Geometry: final body of the model. Coordinates: model frame, mm. Coordinates: 2 decimals unless noted, no trailing zeros. Order: outer loops, then holes, each group sorted by start corner. A loop starts at its lowest first (then second) coordinate and runs counter-clockwise, first axis right, second up. Notation, with made-up numbers: (-31, -37) -> (1, -37) arc R14 ccw to (1, -11) -> close; hole circle Ø8 at (75.25, 87). An arc over 180 degrees is marked (long way). Answer in a Markdown table with one row per item. Add a question column.
1) Section query B-B on z = -451. Return the cut outline in (x, y).
2) Ray query, line 1 (X direction, y = 12, z = -18); line 2 (X direction, y = 20.2, z = -280); line 3 (Z direction, x = 232, y = 8.75). Return the intervals inside material, ascending. Write a range as from..to.
3) Contact query for flat-ended pins moving along their axis: P1, Ø1.5, axis at y = 6, z = -223.5, coming from the -X side; P2, Ø1.5, axis at y = 6.5, z = 164.5, coming from the +X side; P3, Ø1.5, axis at y = 12.5, z = -389.5, coming from the -X side. Output: stop coordinate, or through.
4) Section query A-A on x = -241. Return the cut outline in (y, z), then the cut area to 3 significant figures.
```python
from build123d import *

# Parameters (mm, degrees)
ESQUISSE1_R             = 600
BOSS_EXTRU_1_DEPTH      = 22
ESQUISSE2_R             = 4
ENL_V_MAT_EXTRU_1_DEPTH = 23
ENL_V_MAT_EXTRU_2_DEPTH = 8
ESQUISSE4_R             = 12
ENL_V_MAT_EXTRU_3_DEPTH = 5
ESQUISSE6_R             = 3
ENL_V_MAT_EXTRU_4_DEPTH = 23


with BuildPart() as part:
    # Esquisse1 → Boss.-Extru.1 (new body)
    with BuildSketch(Plane(origin=(0, 0, 0), x_dir=(1, 0, 0), z_dir=(0, 1, 0))):
        with Locations(Location((0, 0, 0), (0, 0, 270))):  # turned: the seam where the file's is
            Circle(ESQUISSE1_R)
    extrude(amount=BOSS_EXTRU_1_DEPTH)

    # Esquisse2 → Enlèv. mat.-Extru.1 (cut, through all)
    with BuildSketch(Plane(origin=(0, 22, 0), x_dir=(1, 0, 0), z_dir=(0, 1, 0))):
        with Locations(Location((0, 280, 0), (0, 0, 270))):  # turned: the seam where the file's is
            Circle(ESQUISSE2_R)
    extrude(amount=-ENL_V_MAT_EXTRU_1_DEPTH, mode=Mode.SUBTRACT)

    # Esquisse3 → Enlèv. mat.-Extru.2 (cut)
    with BuildSketch(Plane.XZ):
        Polygon((6.5, -280), (6.5, -276.24722325), (3.25, -274.370834875), (0, -272.494446501), (-3.25, -274.370834875), (-6.5, -276.24722325), (-6.5, -280), (-6.5, -283.75277675), (-3.25, -285.629165125), (0, -287.505553499), (3.25, -285.629165125), (6.5, -283.75277675), align=None)
    extrude(amount=-ENL_V_MAT_EXTRU_2_DEPTH, mode=Mode.SUBTRACT)

    # Esquisse4 → Enlèv. mat.-Extru.3 (cut)
    with BuildSketch(Plane(origin=(0, 22, 0), x_dir=(1, 0, 0), z_dir=(0, 1, 0))):
        with Locations(Location((0, 280, 0), (0, 0, 270))):  # turned: the seam where the file's is
            Circle(ESQUISSE4_R)
    extrude(amount=-ENL_V_MAT_EXTRU_3_DEPTH, mode=Mode.SUBTRACT)

    # Esquisse6 → Enlèv. mat.-Extru.4 (cut, through all)
    with BuildSketch(Plane(origin=(0, 22, 0), x_dir=(1, 0, 0), z_dir=(0, 1, 0))):
        with Locations(Location((-27.359707791, 541.773153337, 0), (0, 0, 270))):  # turned: the seam where the file's is
            Circle(ESQUISSE6_R)
        with Locations(Location((-27.359707791, 531.883070045, 0), (0, 0, 270))):  # turned: the seam where the file's is
            Circle(ESQUISSE6_R)
        with Locations(Location((-17.338422342, 531.883070045, 0), (0, 0, 270))):  # turned: the seam where the file's is
            Circle(ESQUISSE6_R)
        with Locations(Location((-27.359707791, 589.516341352, 0), (0, 0, 270))):  # turned: the seam where the file's is
            Circle(ESQUISSE6_R)
        with Locations(Location((-27.359707791, 573.664786381, 0), (0, 0, 270))):  # turned: the seam where the file's is
            Circle(ESQUISSE6_R)
        with Locations(Location((-17.338422342, 589.516341352, 0), (0, 0, 270))):  # turned: the seam where the file's is
            Circle(ESQUISSE6_R)
        with Locations(Location((17.587577233, 589.516341352, 0), (0, 0, 270))):  # turned: the seam where the file's is
            Circle(ESQUISSE6_R)
        with Locations(Location((29.13602426, 589.516341352, 0), (0, 0, 270))):  # turned: the seam where the file's is
            Circle(ESQUISSE6_R)
        with Locations(Location((29.13602426, 573.664786381, 0), (0, 0, 270))):  # turned: the seam where the file's is
            Circle(ESQUISSE6_R)
        with Locations(Location((29.13602426, 541.773153337, 0), (0, 0, 270))):  # turned: the seam where the file's is
            Circle(ESQUISSE6_R)
        with Locations(Location((29.13602426, 531.883070045, 0), (0, 0, 270))):  # turned: the seam where the file's is
            Circle(ESQUISSE6_R)
        with Locations(Location((17.587577233, 531.883070045, 0), (0, 0, 270))):  # turned: the seam where the file's is
            Circle(ESQUISSE6_R)
    extrude(amount=-ENL_V_MAT_EXTRU_4_DEPTH, mode=Mode.SUBTRACT)


solid = part.part
```
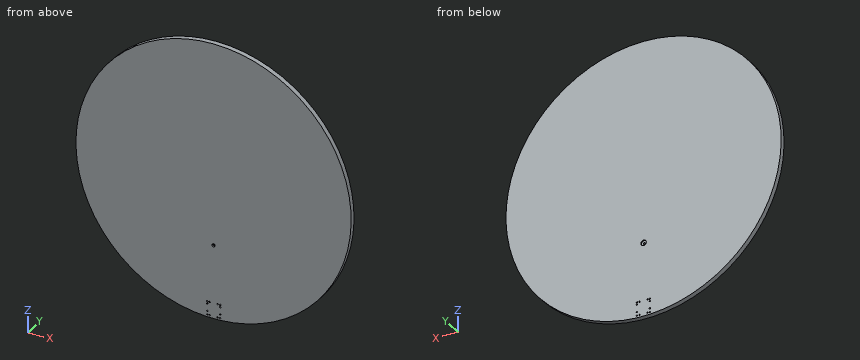
Result:
| question | item | result |
|---|---|---|
| 1 | outline | (-395.73, 0) -> (395.73, 0) -> (395.73, 22) -> (-395.73, 22) -> close |
| 2 | line 1 | -599.73..599.73 |
| 2 | line 2 | -530.66..-12, 12..530.66 |
| 2 | line 3 | -553.33..553.33 |
| 3 | P1 | x = -557.12 |
| 3 | P2 | x = 577.22 |
| 3 | P3 | x = -457.03 |
| 4 | outline | (0, -549.47) -> (22, -549.47) -> (22, 549.47) -> (0, 549.47) -> close |
| 4 | area | 24,200 mm2 |
